```python
from build123d import *

# Parameters (mm, degrees)
F0_W      = 111.984528
F0_H      = 85.756578
F1_DEPTH  = 3
F2_W      = 6.280169
F2_H      = 6.403141
F2_W_2    = 99.42419
F2_H_2    = 79.353437
F3_DEPTH  = 50.8
F4_W      = 14.75576
F4_H      = 16.726847
F5_DEPTH  = 25.4
F6_W      = 15.188249
F6_H      = 15.062956
F7_DEPTH  = 15
F9_W      = 14.695715
F9_H      = 14.967857
F9_W_2    = 15.512146
F9_H_2    = 15.784284
F10_DEPTH = 15


with BuildPart() as f1:
    # F0 (on Top) → F1 (new body)
    with BuildSketch(Plane.XY):
        Rectangle(F0_W, F0_H)
    extrude(amount=F1_DEPTH)

    # F2 (on face) → F3 (join)
    with BuildSketch(Plane.XY.offset(3)):
        with Locations((-52.852179, 39.676718)):
            Rectangle(F2_W, F2_H)
        with Locations((0, 39.676718)):
            Rectangle(F2_W_2, F2_H)
        with Locations((-52.852179, -3.20157)):
            Rectangle(F2_W, F2_H_2)
        with Locations((52.852179, 39.676718)):
            Rectangle(F2_W, F2_H)
        with Locations((52.852179, -3.20157)):
            Rectangle(F2_W, F2_H_2)
    extrude(amount=F3_DEPTH)

    # F4 (on face) → F5 (cut)
    with BuildSketch(Plane.YZ.offset(55.992264)):
        with Locations((26.207732, 38.103093)):
            Rectangle(F4_W, F4_H)
    extrude(amount=-F5_DEPTH, mode=Mode.SUBTRACT)

    # F6 (on face) → F7 (join)
    with BuildSketch(Plane.XY.offset(3)):
        with Locations((7.594124, 28.94367)):
            Rectangle(F6_W, F6_H)
    extrude(amount=F7_DEPTH)

    # F9 (on face) → F10 (join)
    with BuildSketch(Plane.XY.offset(3)):
        with Locations((-42.454285, 29.255357)):
            Rectangle(F9_W, F9_H)
        with Locations((41.773926, 28.847144)):
            Rectangle(F9_W_2, F9_H_2)
    extrude(amount=F10_DEPTH)


solid = f1.part
```
Model file for the job. Use its own axes, mm. A direction names the side the tool comes from. Give positions to 0.01 mm unless a question says otherwise; leave off trailing zeros. Loops run counter-clockwise (first coordinate to the right, second up) from the corner with the lowest first, then second, coordinate; pieces in that order, holes last. Notation, with made-up numbers: (10, 38.25) - (16, 38.25) arc R18 ccw to (16, 59.25) - close; hole circle Ø7 at (71.25, 48). An arc over 180 degrees is marked (long way). One line per item, written item: value. Start each with the question number.
1. Slice it at B-B (x = 17.5). List the corners of the cut face in (y, z), plus the area to 3 significant figures.
2. Which spindle directions (+Z, -Z, +X, -X, +Y, -Y) get a long thin tool onto all of the face, cutting with end or side? Do faces 5 (the flat face through (-55.992, -1, 1)), 6 (the flat face through (53, 26, 46.467)), 7 (the flat face through (-49.712, -4, 28)). Say none if no direction does.
3. Probe L1, parallel to X at y = -6, z = 33.5; L2, parallel to Z at x = 30, y = -10.5; L3, parallel to Y at x = -6.5, z = 19.5. List the from-to ranges inside material, lowest first. Write a range as from..to.
4. Pull direction Y, two halves, no side cores. Call faces 1 (the flat face through (42, 29, 18)), 2 (the flat face through (53, 26, 29.74)), 3 (the flat face through (-1, 42.878, 1)), 4 (the flat face through (53, 33.586, 38)): pulls with the +Y half, pulls with the -Y half, needs draft (parallel to the pull), parting line crosses it, or undercut.
5. Slice it at A-A (z = 4.5). List the corners of the cut face in (x, y) (3 decimals), plus the area to 3 significant figures.
6. Slice it at D-D (y = 13.5). List the corners of the cut face in (x, z).
7. Slice it at C-C (y = 31.5). List the corners of the cut face in (x, z), plus the area to 3 significant figures.
8. Pin check, flat tips, straight feed: pin 1 (8 mm diameter, centred on x = -25, y = 23, fed in from +Z); pin 2 (11.5 mm diameter, centred on x = -44, z = 7, fed in from -Y); pin 3 (7.5 mm diameter, centred on x = 5, y = 26.5, fed in from +Z); pin 4 (12 mm diameter, centred on x = 5, z = 9.5, fed in from -Y). Stop position of each tip, or through.
Solution:
1. outline: (-42.88, 0) - (42.88, 0) - (42.88, 53.8) - (36.48, 53.8) - (36.48, 3) - (-42.88, 3) - close
1. area: 583 mm^2
2. face 5: +Z, -Z, -X, +Y, -Y
2. face 6: +X
2. face 7: +Z, -Y
3. L1: x = -55.99..-49.71, 49.71..55.99
3. L2: z = 0..3
3. L3: y = 36.48..42.88
4. face 1: needs draft
4. face 2: undercut
4. face 3: pulls with the +Y half
4. face 4: undercut
5. outline: (-55.992, -42.878) - (-49.712, -42.878) - (-49.712, 21.771) - (-35.106, 21.771) - (-35.106, 36.475) - (0, 36.475) - (0, 21.412) - (15.188, 21.412) - (15.188, 36.475) - (34.018, 36.475) - (34.018, 20.955) - (49.53, 20.955) - (49.53, 36.475) - (49.712, 36.475) - (49.712, -42.878) - (55.992, -42.878) - (55.992, 42.878) - (-55.992, 42.878) - close
5. area: 2,400 mm^2
6. outline: (-55.99, 0) - (55.99, 0) - (55.99, 53.8) - (49.71, 53.8) - (49.71, 3) - (-49.71, 3) - (-49.71, 53.8) - (-55.99, 53.8) - close
7. outline: (-55.99, 0) - (55.99, 0) - (55.99, 29.74) - (49.71, 29.74) - (49.71, 3) - (49.53, 3) - (49.53, 18) - (34.02, 18) - (34.02, 3) - (15.19, 3) - (15.19, 18) - (0, 18) - (0, 3) - (-35.11, 3) - (-35.11, 18) - (-49.71, 18) - (-49.71, 53.8) - (-55.99, 53.8) - close; (49.71, 46.47) - (55.99, 46.47) - (55.99, 53.8) - (49.71, 53.8) - close
7. area: 1,550 mm^2
8. pin 1: stops at z = 3
8. pin 2: stops at y = -42.88
8. pin 3: stops at z = 18
8. pin 4: stops at y = 21.41
